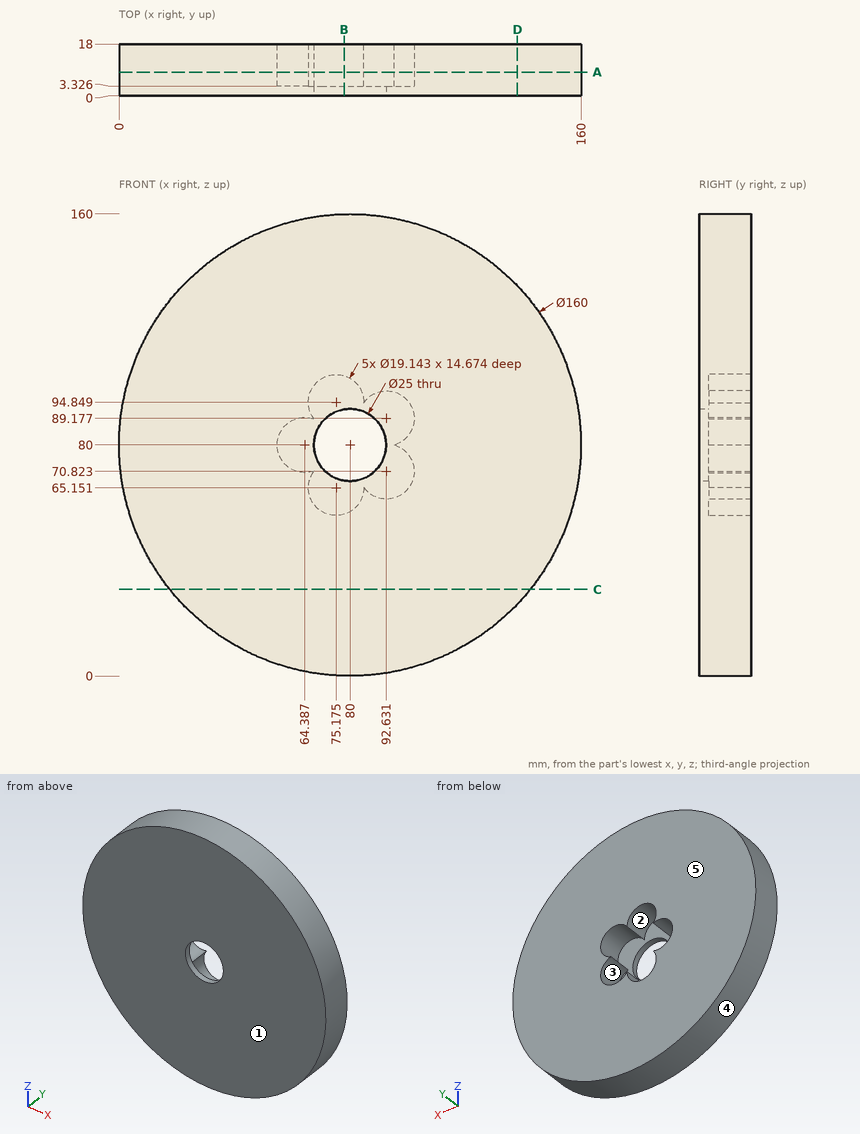
Design review of the part shown in the three views and the two pictorial views. Dimensions are in mm from the part's minimum x, y and z. A direction names the side the tool comes from. Coordinates: 2 decimals unless noted, no trailing zeros. Loops run counter-clockwise (first coordinate to the right, second up) from the corner with the lowest first, then second, coordinate; pieces in that order, holes last.
(1) Consider section A-A, the plane y = 8.25. Give the boundary of the cut face in (x, z) (1 decimal).
Determined:
outline: circle Ø160 at (80, 80); hole (67.6, 71) arc R9.6 ccw (long way) to (84.7, 65.4) arc R9.6 ccw (long way) to (95.4, 80) arc R9.6 ccw (long way) to (84.7, 94.6) arc R9.6 ccw (long way) to (67.6, 89) arc R9.6 ccw (long way) to start
(2) Consider section D-D, the plane x = 138. Give the boundary of the cut face in (y, z), plus the area to 3 significant figures.
Determined:
outline: (0, 24.9) - (18, 24.9) - (18, 135.1) - (0, 135.1) - close
area: 1,980 mm2
(3) Tool access review of the marked faces 1 and 2: name each direction out of +Z, -Z, +X, -X, +Y, -Y from which nothing blocks a thin tool from reaching the whole face with its end or side.
Determined:
face 1: +Z, -Z, +X, -X, -Y
face 2: +Y
(4) Consider section C-C, the plane z = 30. Give the boundary of the cut face in (x, y), plus the area to 3 significant figures.
Determined:
outline: (17.55, 0) - (142.45, 0) - (142.45, 18) - (17.55, 18) - close
area: 2,250 mm2
(5) Draft analysis for pull direction Z (two halves, no side actions). For the marked faces 3, 4 and 5, state which applies: +Z half, -Z half, draft (parallel to the pull), parting line (faces both ways), or undercut.
Determined:
face 3: undercut
face 4: parting line
face 5: draft
(6) Insertion check: P1, Ø11.5, axis at x = 75.18, z = 94.85, coming from the +Y side; P2, Ø4, axis at x = 118.5, y = 10, coming from the -Z side; P3, Ø1, axis at y = 9, z = 86, coming from the +X side. Each pin has a flat end and moves straight along its axis. Give the tip position at first contact, or say it passes through.
Determined:
P1: stops at y = 3.33
P2: stops at z = 8.81
P3: stops at x = 159.81
(7) Wall thickness on L1, parallel to X at y = 1.45, z = 80; L2, parallel to X at y = 16.25, z = 86 (1 decimal); L3, parallel to Z at x = 75.5, y = 5 (1 decimal): over which ranges is each line inside the solid? List them lowest first.
Determined:
L1: x = 0 to 67.5, 92.5 to 160
L2: x = 0.2 to 56.9, 101.7 to 159.8
L3: z = 0.1 to 55.6, 104.4 to 159.9
(8) Consider section B-B, the plane x = 78. Give the boundary of the cut face in (y, z) (1 decimal).
Determined:
outline: (0, 0) - (18, 0) - (18, 56) - (3.3, 56) - (3.3, 67.7) - (0, 67.7) - close; (0, 92.3) - (3.3, 92.3) - (3.3, 104) - (18, 104) - (18, 160) - (0, 160) - close
